For this review, take the finished solid that the model builds, in its own axes (mm). A direction names the side the tool comes from. Coordinates: 2 decimals unless noted, no trailing zeros. Write each loop counter-clockwise with the first axis right and the second up, starting at its lowest first coordinate (ties: lowest second). Pieces come first, ordered by that corner, then holes. Notation, with made-up numbers: M 46.25,12 L 59.25,12 A15 cw 59.25,29 Z; hole C 45,79.25 d8. An arc over 180 degrees is marked long. Return JSON: item names as keys, results as strings.
```python
from build123d import *

# Parameters (mm, degrees)
ESQUISSE1_R        = 4
BOSS_EXTRU_1_DEPTH = 10
ESQUISSE2_R        = 5
BOSS_EXTRU_2_DEPTH = 80
ESQUISSE3_R        = 4
BOSS_EXTRU_3_DEPTH = 10
CHANFREIN1_SIZE    = 0.5


with BuildPart() as part:
    # Esquisse1 → Boss.-Extru.1 (new body)
    with BuildSketch(Plane.XY):
        Circle(ESQUISSE1_R)
    extrude(amount=BOSS_EXTRU_1_DEPTH)

    # Esquisse2 → Boss.-Extru.2 (add)
    with BuildSketch(Plane.XY.offset(10)):
        Circle(ESQUISSE2_R)
    extrude(amount=BOSS_EXTRU_2_DEPTH)

    # Esquisse3 → Boss.-Extru.3 (add)
    with BuildSketch(Plane.XY.offset(90)):
        Circle(ESQUISSE3_R)
    extrude(amount=BOSS_EXTRU_3_DEPTH)

    # Chanfrein1
    chanfrein1_edges = [part.edges().sort_by_distance(p)[0] for p in [
        (-4, 0, 100),
        (-4, 0, 0),
    ]]
    chamfer(chanfrein1_edges, length=CHANFREIN1_SIZE)


solid = part.part
```
1. We need section A-A (y = 0). State the section outline as (x, z) points.
Checks:
{"outline": "M -5,10 L -4,10 L -4,0.5 L -3.5,0 L 3.5,0 L 4,0.5 L 4,10 L 5,10 L 5,90 L 4,90 L 4,99.5 L 3.5,100 L -3.5,100 L -4,99.5 L -4,90 L -5,90 Z"}
2. Clearance check with flat-ended pins moving along their axes: pin 1 Ø3 at (y, z) = (2.5, 70.5) entering from -X; pin 2 Ø4 at (x, z) = (1.5, 77.5) entering from -Y; pin 3 Ø3 at (y, z) = (-3.5, 16.5) entering from -X; pin 4 Ø1.5 at (x, y) = (4, 2.5) entering from +Z. State where each tip first meets the part, or that it passes through.
Checks:
{"pin 1": "x = -4.9", "pin 2": "y = -5", "pin 3": "x = -4.58", "pin 4": "z = 99.53"}
3. We need section C-C (z = 27.5). State the section outline as (x, y) points, plus the area to 3 significant figures.
Checks:
{"outline": "C 0,0 d10", "area": "78.5 mm2"}
4. For faces 1 (the face through (-0.867, -3.905, 5.184)), 2 (the face through (-0.867, -3.905, 94.684)), 3 (the face through (0, 0, 0)), list the 3-axis set-ups (+Z, -Z, +X, -X, +Y, -Y) from which the entire face can be reached by the end or side of a thin tool; tool diameter is ignored.
Checks:
{"face 1": "-Z", "face 2": "+Z", "face 3": "-Z, +X, -X, +Y, -Y"}
5. Wall thickness on L1, parallel to Z at x = -3.75, y = -1.5; L2, parallel to X at y = -0.25, z = 11; L3, parallel to X at y = 3, z = 71.5: over which ranges is each line inside the solid? List them lowest first. Write a range as from..to.
Checks:
{"L1": "10..90", "L2": "-4.99..4.99", "L3": "-4..4"}
